from build123d import *

# Parameters (mm, degrees)
BOSS_EXTRUDE1_DEPTH      = 4
BOSS_EXTRUDE1_DEPTH_BACK = 5.8
SKETCH1_W                = 11
SKETCH1_H                = 5
SKETCH1_R                = 0.975
SKETCH1_W_2              = 5.75
SKETCH1_H_2              = 2.85
CUT_EXTRUDE1_DEPTH       = 10.901799079
CUT_EXTRUDE1_DEPTH_BACK  = 10.901799079
SKETCH3_W                = 3
SKETCH3_H                = 4
SKETCH4_W                = 1.375
SKETCH4_H                = 2.85
BOSS_EXTRUDE3_DEPTH      = 1
FILLET1_R                = 0.3
FILLET2_R                = 0.3


with BuildPart() as part:
    # Sketch1 → Boss-Extrude1 (new, two sides: drawn at the far end of the back side and taken through both)
    with BuildSketch(Plane.XY.offset(-BOSS_EXTRUDE1_DEPTH_BACK)):
        with Locations((1.5, -1.325)):
            Rectangle(SKETCH1_W, SKETCH1_H)
        with Locations((5, -1.325)):
            Circle(SKETCH1_R, mode=Mode.SUBTRACT)
        with Locations((0, -1.325)):
            Rectangle(SKETCH1_W_2, SKETCH1_H_2, mode=Mode.SUBTRACT)
    extrude(amount=BOSS_EXTRUDE1_DEPTH + BOSS_EXTRUDE1_DEPTH_BACK)

    # Sketch3 → Cut-Extrude1 (cut, two sides: drawn at the far end of the back side and taken through both)
    with BuildSketch(Plane(origin=(0, -2.75, 0), x_dir=(1, 0, 0), z_dir=(0, 1, 0)).offset(-CUT_EXTRUDE1_DEPTH_BACK)):
        with Locations((0, 3.8)):
            Rectangle(SKETCH3_W, SKETCH3_H)
    extrude(amount=CUT_EXTRUDE1_DEPTH + CUT_EXTRUDE1_DEPTH_BACK, mode=Mode.SUBTRACT)

    # Sketch4 → Boss-Extrude3 (add)
    with BuildSketch(Plane(origin=(0, 0, -5.8), x_dir=(-1, 0, 0), z_dir=(0, 0, -1))):
        with Locations((-2.1875, -1.325)):
            Rectangle(SKETCH4_W, SKETCH4_H)
        with Locations((2.1875, -1.325)):
            Rectangle(SKETCH4_W, SKETCH4_H)
    extrude(amount=-BOSS_EXTRUDE3_DEPTH)

    # Fillet1
    fillet1_edges = [part.edges().sort_by_distance(p)[0] for p in [
        (-4, 1.175, -0.9),
        (7, 1.175, -0.9),
        (7, -3.825, -0.9),
        (-4, -3.825, -0.9),
    ]]
    fillet(fillet1_edges, radius=FILLET1_R)

    # Fillet2
    fillet2_edges = [part.edges().sort_by_distance(p)[0] for p in [
        (-2.6, 1.175, -5.8),
        (4.1, -3.825, -5.8),
        (7, -1.325, -5.8),
        (6.912132034, -3.737132034, -5.8),
        (6.912132034, 1.087132034, -5.8),
        (-4, -1.325, -5.8),
        (-3.912132034, 1.087132034, -5.8),
        (-3.912132034, -3.737132034, -5.8),
        (4.025, -1.325, -5.8),
        (4.1, 1.175, -5.8),
        (-2.6, -3.825, -5.8),
        (1.5, -1.325, -5.8),
        (-1.5, -1.325, -5.8),
    ]]
    fillet(fillet2_edges, radius=FILLET2_R)


solid = part.part
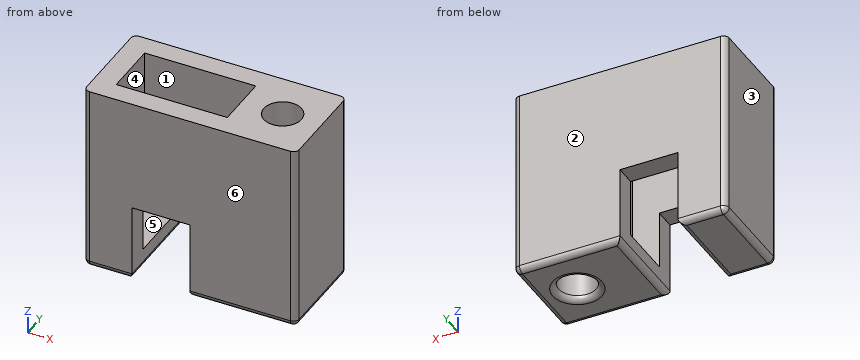
Work out the finished part from the listing and answer in its coordinate system (mm). Face numbers are marked on the shaded views. A direction names the side the tool comes from. Give positions to 0.01 mm unless a question says otherwise; leave off trailing zeros. Loops run counter-clockwise (first coordinate to the right, second up) from the corner with the lowest first, then second, coordinate; pieces in that order, holes last. Notation, with made-up numbers: (-24, -19) - (35, -19) arc R36 ccw to (35, 15) - close; hole circle Ø1 at (-33.5, 13). An arc over 180 degrees is marked (long way). Answer in a Markdown table with one row per item.
(1) A flat-ended cylindrical pin translates along its axis: pin 1 Ø0.9 at (x, y) = (0, 0.5) entering from -Z. Find the tip coordinate at first contact, or state that the pin passes through.
Results list:
| item | result |
|---|---|
| pin 1 | stops at z = -1.8 |
(2) For a pull along Y with two mould halves and no side action, classify the marked faces 1, 2, 3 and 4 as pulls with the +Y half, pulls with the -Y half, needs draft (parallel to the pull), parting line crosses it, or undercut.
Results list:
| item | result |
|---|---|
| face 1 | undercut |
| face 2 | pulls with the +Y half |
| face 3 | needs draft |
| face 4 | undercut |
(3) Section B-B (z = 0) is taken. Give the vertices of the cut face in (x, y) (3 decimals), and give its area (3 significant figures).
Results list:
| item | result |
|---|---|
| outline | (-4, -3.525) arc R0.3 ccw to (-3.7, -3.825) - (6.7, -3.825) arc R0.3 ccw to (7, -3.525) - (7, 0.875) arc R0.3 ccw to (6.7, 1.175) - (-3.7, 1.175) arc R0.3 ccw to (-4, 0.875) - close; hole (-2.875, -2.75) - (2.875, -2.75) - (2.875, 0.1) - (-2.875, 0.1) - close; hole circle Ø1.95 at (5, -1.325) |
| area | 35.5 mm² |
(4) A tool of negligible diameter and unlimited length cuts with its end or side. For the marked faces 5 and 6, from which of +Z, -Z, +X, -X, +Y, -Y can it reach the whole face along a straight path? Write none if from no direction.
Results list:
| item | result |
|---|---|
| face 5 | +Z |
| face 6 | +Z, -Z, +X, -X, -Y |
(5) Section D-D (x = 2) is taken. Give the vertices of the cut face in (y, z) (3 decimals).
Results list:
| item | result |
|---|---|
| outline | (-3.825, -5.5) arc R0.3 ccw to (-3.525, -5.8) - (0.875, -5.8) arc R0.3 ccw to (1.175, -5.5) - (1.175, 4) - (0.1, 4) - (0.1, -4.8) - (-2.75, -4.8) - (-2.75, 4) - (-3.825, 4) - close |
(6) Section A-A (x = 5) is taken. Give the vertices of the cut face in (y, z) (3 decimals), and give its area (3 significant figures).
Results list:
| item | result |
|---|---|
| outline | (-3.825, -5.5) arc R0.3 ccw to (-3.525, -5.8) - (-2.6, -5.8) arc R0.3 ccw to (-2.3, -5.5) - (-2.3, 4) - (-3.825, 4) - close; (-0.35, -5.5) arc R0.3 ccw to (-0.05, -5.8) - (0.875, -5.8) arc R0.3 ccw to (1.175, -5.5) - (1.175, 4) - (-0.35, 4) - close |
| area | 29.8 mm² |
(7) Section C-C (y = -3.1) is taken. Give the vertices of the cut face in (x, z), and give its area (3 significant figures).
Results list:
| item | result |
|---|---|
| outline | (-4, -5.5) arc R0.3 ccw to (-3.7, -5.8) - (-1.8, -5.8) arc R0.3 ccw to (-1.5, -5.5) - (-1.5, -1.8) - (1.5, -1.8) - (1.5, -5.5) arc R0.3 ccw to (1.8, -5.8) - (6.7, -5.8) arc R0.3 ccw to (7, -5.5) - (7, 4) - (-4, 4) - close |
| area | 95.7 mm² |
(8) Consider L1, parallel to X at y = -3.1, z = -4; L2, parallel to X at y = -2.1, z = -0.25 (3 decimals); L3, parallel to Y at x = 5, z = -3.5 (3 decimals). Determine where each line is inside the solid, lowest interval first. Write a range as [from, to].
Results list:
| item | result |
|---|---|
| L1 | x = [-4, -1.5], [1.5, 7] |
| L2 | x = [-4, -2.875], [2.875, 4.408], [5.592, 7] |
| L3 | y = [-3.825, -2.3], [-0.35, 1.175] |
